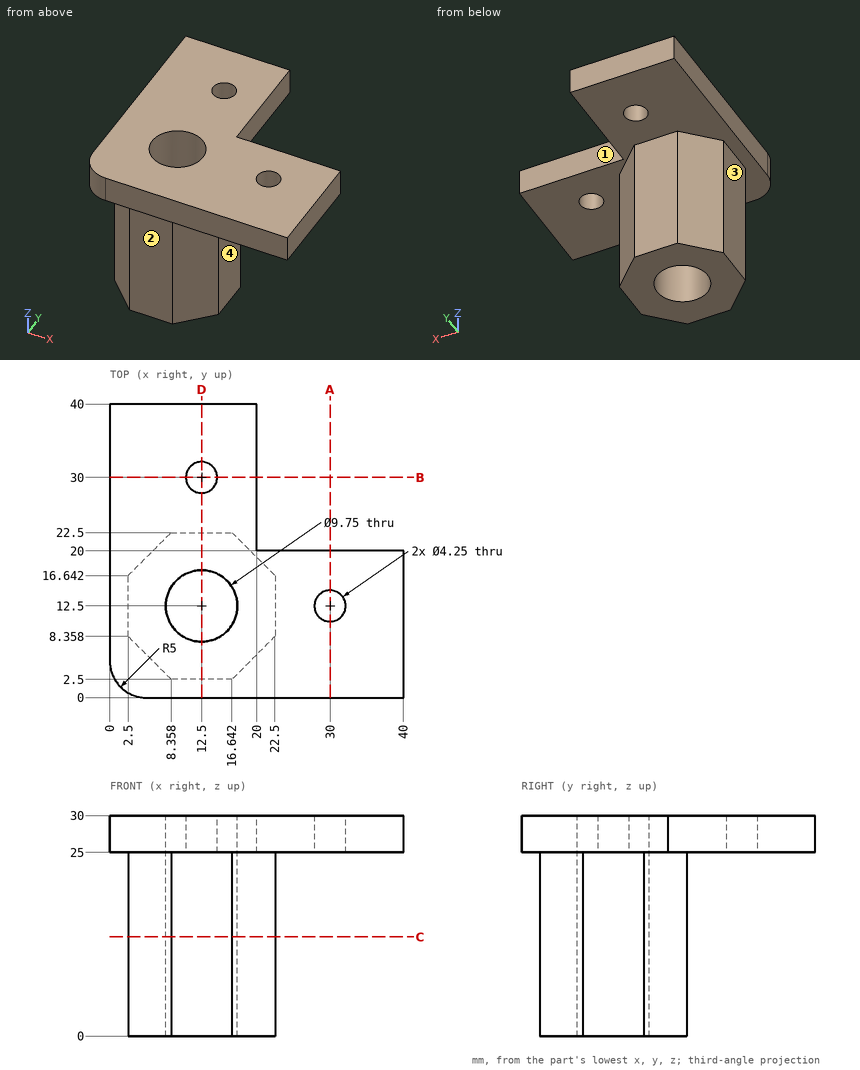
Geometry check sheet. Reference: drawing and pictorial views, mm from the part's lowest x, y, z. A direction names the side the tool comes from. Round coordinates to 2 decimals unless told otherwise and drop trailing zeros. Loops run counter-clockwise (first coordinate to the right, second up) from the corner with the lowest first, then second, coordinate; pieces in that order, holes last. Notation, with made-up numbers: (85.25, 59.25) -> (136.25, 59.25) arc R19 cw to (136.25, 88.25) -> close; hole circle Ø4 at (60, -19.5). An arc over 180 degrees is marked (long way). Answer as a JSON object with one key per item and string values. Group by question number.
Item 1: Cross-section at D-D, the plane x = 12.5. Record the cut outline in (y, z) (3 decimals).
Item 2: Thickness scan on line 1 along Y through (x, z) = (12.5, 28.4) (3 decimals); line 2 along Y through (x, z) = (12.5, 13.75) (3 decimals); line 3 along Y through (x, z) = (30, 27.6) (3 decimals). Record the ranges inside material, lowest first.
Item 3: Depth check by flat-ended pin: pin 1 Ø12 at (x, y) = (26.5, 25) entering from -Z; pin 2 Ø12 at (x, z) = (24.5, 12.5) entering from -Y; pin 3 Ø9 at (y, z) = (11, 8.5) entering from +X. Enter the tip coordinate at first touch or a pass-through.
Item 4: Cross-section at C-C, the plane z = 13.5. Record the cut outline in (x, y) (3 decimals).
Item 5: Cross-section at A-A, the plane x = 30. Record the cut outline in (y, z) (3 decimals).
Item 6: Set-up check for the marked faces 1, 2, 3 and 4: record each of +Z, -Z, +X, -X, +Y, -Y from which the full face is reachable in a straight line by a thin tool's end or side.
Determined:
{
 "1": {"outline": "(0, 25) -> (2.5, 25) -> (2.5, 0) -> (7.625, 0) -> (7.625, 30) -> (0, 30) -> close; (17.375, 0) -> (22.5, 0) -> (22.5, 25) -> (27.875, 25) -> (27.875, 30) -> (17.375, 30) -> close; (32.125, 25) -> (40, 25) -> (40, 30) -> (32.125, 30) -> close"},
 "2": {"line 1": "y = 0 to 7.625, 17.375 to 27.875, 32.125 to 40", "line 2": "y = 2.5 to 7.625, 17.375 to 22.5", "line 3": "y = 0 to 10.375, 14.625 to 20"},
 "3": {"pin 1": "stops at z = 25", "pin 2": "stops at y = 4.36", "pin 3": "stops at x = 22.5"},
 "4": {"outline": "(2.5, 8.358) -> (8.358, 2.5) -> (16.642, 2.5) -> (22.5, 8.358) -> (22.5, 16.642) -> (16.642, 22.5) -> (8.358, 22.5) -> (2.5, 16.642) -> close; hole circle Ø9.75 at (12.5, 12.5)"},
 "5": {"outline": "(0, 25) -> (10.375, 25) -> (10.375, 30) -> (0, 30) -> close; (14.625, 25) -> (20, 25) -> (20, 30) -> (14.625, 30) -> close"},
 "6": {"face 1": "+Z, -Z, +X, +Y", "face 2": "-Z, +X, -X, -Y", "face 3": "-Z, -X, +Y, -Y", "face 4": "-Z, +X, +Y, -Y"}
}
